```python
from build123d import *

# Parameters (mm, degrees)
SKETCH1_R           = 3.875
BOSS_EXTRUDE1_DEPTH = 34.78
SKETCH2_OUTSIDE_W   = 17.044
SKETCH2_OUTSIDE_H   = 17.044
SKETCH2_OUTSIDE_R   = 2.39
CUT_EXTRUDE1_DEPTH  = 30
CHAMFER1_SIZE       = 0.5
CUT_EXTRUDE2_DEPTH  = 3.36


with BuildPart() as part:
    # Sketch1 → Boss-Extrude1 (new body)
    with BuildSketch(Plane(origin=(0, 0, 0), x_dir=(1, 0, 0), z_dir=(0, 1, 0))):
        Circle(SKETCH1_R)
    extrude(amount=BOSS_EXTRUDE1_DEPTH)

    # Sketch2 outside → Cut-Extrude1 (cut)
    with BuildSketch(Plane(origin=(0, 34.78, 0), x_dir=(1, 0, 0), z_dir=(0, 1, 0))):
        Rectangle(SKETCH2_OUTSIDE_W, SKETCH2_OUTSIDE_H)
        Circle(SKETCH2_OUTSIDE_R, mode=Mode.SUBTRACT)
    extrude(amount=-CUT_EXTRUDE1_DEPTH, mode=Mode.SUBTRACT)

    # Chamfer1
    chamfer1_edges = [part.edges().sort_by_distance(p)[0] for p in [
        (-2.39, 34.78, 0),
    ]]
    chamfer(chamfer1_edges, length=CHAMFER1_SIZE)

    # Sketch8 → Cut-Extrude2 (cut)
    with BuildSketch(Plane.XZ):
        Polygon((2.644264233, 0), (1.322132116, 2.29), (-1.322132116, 2.29), (-2.644264233, 0), (-1.322132116, -2.29), (1.322132116, -2.29), align=None)
    extrude(amount=-CUT_EXTRUDE2_DEPTH, mode=Mode.SUBTRACT)


solid = part.part
```
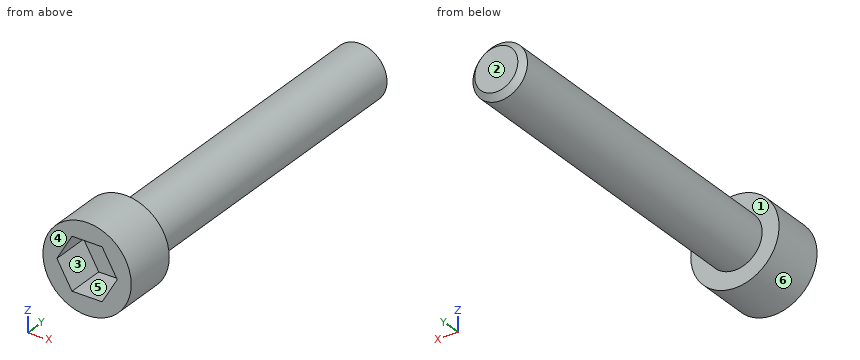
Could you check a few things on this model? Use its own coordinates, in mm. Face numbers are marked on the shaded views. A direction names the side the tool comes from. Round coordinates to 2 decimals unless told otherwise and drop trailing zeros. Write each loop counter-clockwise with the first axis right and the second up, starting at its lowest first coordinate (ties: lowest second). Pieces come first, ordered by that corner, then holes. Notation, with made-up numbers: M -32.75,-8 L -6.75,-8 A23 cw -6.75,29 Z; hole C -3.75,43 d11. An arc over 180 degrees is marked long. Answer in a Markdown table with one row per item. Add a question column.
Q1. Imagine slicing it at D-D (y = 4). Please give me the cut outline in (x, z) (3 decimals).
Q2. If I drill on line 1 (Y direction, x = -1.5, z = -3.5); line 2 (Z direction, x = -1, y = 3); line 3 (Y direction, x = -1.75, z = -0.25), over which ranges is the centre line in solid material (lowest first)? Write a range as from..to.
Q3. Imagine slicing it at C-C (z = -3.5). Please give me the cut outline in (x, y).
Q4. Imagine slicing it at A-A (x = 0). Please give me the cut outline in (y, z) (3 decimals), then the cut area to 3 significant figures.
Q5. On a 3-axis mill with a long thin cutter (end or side, diameter ignored), from which of +Z, -Z, +X, -X, +Y, -Y can I reach the whole of each face in a straight line? I mean the marked faces 1 and 2. Say none if no direction works.
Q6. Imagine slicing it at B-B (y = 11.5). Please give me the cut outline in (x, z).
Q7. Will these pins go through, and if not, where does the flat tip stop? pin 1 Ø4 at (x, y) = (3, 22) entering from +Z; pin 2 Ø1.5 at (y, z) = (14.5, 0) entering from +X; pin 3 Ø1.5 at (y, z) = (21.5, 2.5) entering from +X.
Q8. If we mould it in two halves opening along Z, with no side actions, what happens to the marked faces 3, 4, 5 and 6? For each: +Z half, -Z half, draft (parallel to the pull), parting line (faces both ways), or undercut.
Values:
| question | item | result |
|---|---|---|
| 1 | outline | C 0,0 d7.75 |
| 2 | line 1 | 0..4.78 |
| 2 | line 2 | -3.74..-2.29, 2.29..3.74 |
| 2 | line 3 | 3.36..34.78 |
| 3 | outline | M -1.66,0 L 1.66,0 L 1.66,4.78 L -1.66,4.78 Z |
| 4 | outline | M 0,-3.875 L 4.78,-3.875 L 4.78,-2.39 L 34.28,-2.39 L 34.78,-1.89 L 34.78,1.89 L 34.28,2.39 L 4.78,2.39 L 4.78,3.875 L 0,3.875 L 0,2.29 L 3.36,2.29 L 3.36,-2.29 L 0,-2.29 Z |
| 4 | area | 165 mm^2 |
| 5 | face 1 | +Y |
| 5 | face 2 | +Z, -Z, +X, -X, +Y |
| 6 | outline | C 0,0 d4.78 |
| 7 | pin 1 | z = 2.17 |
| 7 | pin 2 | x = 2.39 |
| 7 | pin 3 | x = 1.63 |
| 8 | face 3 | undercut |
| 8 | face 4 | draft |
| 8 | face 5 | undercut |
| 8 | face 6 | parting line |
